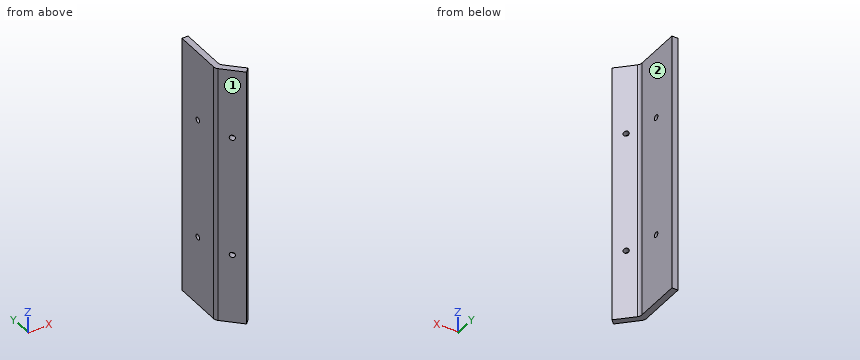
from build123d import *

# Parameters (mm, degrees)
F1_DEPTH = 215
F3_D     = 4.4
F5_D     = 4.4


with BuildPart() as f1:
    # F0 (on Top) → F1 (new body)
    with BuildSketch(Plane.XY):
        with BuildLine():
            Line((0, 2.0710678119), (0, 40))
            Line((0, 40), (-5, 40))
            Line((-5, 40), (-5, 0))
            ThreePointArc((-5, 0), (-4.6193976626, -1.9134171618), (-3.5355339059, -3.5355339059))
            Line((-3.5355339059, -3.5355339059), (10.6066017178, -17.6776695297))
            Line((10.6066017178, -17.6776695297), (14.1421356237, -14.1421356237))
            Line((14.1421356237, -14.1421356237), (1.4644660941, -1.4644660941))
            ThreePointArc((1.4644660941, -1.4644660941), (0.3806023374, 0.15765065), (0, 2.0710678119))
        make_face()
    extrude(amount=F1_DEPTH)

    # F3 (through all)
    with Locations(Plane.YZ):
        with Locations((20, 157.5), (20, 57.5)):
            Hole(F3_D / 2)

    # F5 (through all)
    with Locations(Plane(origin=(0, 0, 0), x_dir=(-0.7071067812, 0.7071067812, 0), z_dir=(0.7071067812, 0.7071067812, 0))):
        with Locations((-10, 157.5), (-10, 57.5)):
            Hole(F5_D / 2)


solid = f1.part
Geometry: final body of the model. Coordinates: model frame, mm. Face numbers are marked on the shaded views. A direction names the side the tool comes from. Round coordinates to 2 decimals unless told otherwise and drop trailing zeros. Loops run counter-clockwise (first coordinate to the right, second up) from the corner with the lowest first, then second, coordinate; pieces in that order, holes last. Notation, with made-up numbers: M 79,61.5 L 107,61.5 A27 cw 107,88.5 Z; hole C 89.25,-22 d9. An arc over 180 degrees is marked long. Put each result on its own line as item: value. Start each with the question number.
(1) Material intervals for line 1 along Z through (x, y) = (-2.6, 20); line 2 along Z through (x, y) = (3.75, -8); line 3 along X through (y, z) = (33, 121), sorted ascending. Write a range as [from, to].
(2) Section query D-D (y = 35.5). Return loops of the section in (x, z), then the cut area to 4 significant figures.
(3) Section query B-B (z = 135.5). Return loops of the section in (x, y).
(4) Contact query for flat-ended pins moving along their axis: pin 1 Ø2 at (x, z) = (6.5, 23.5) entering from -Y; pin 2 Ø1.5 at (x, y) = (-2.5, 6.5) entering from -Z; pin 3 Ø11.5 at (y, z) = (30.5, 135) entering from +X; pin 4 Ø4 at (y, z) = (-3, 179) entering from +X. Output: stop coordinate, or through.
(5) Section query A-A (y = 20). Return loops of the section in (x, z).
(6) Set-up query: the marked faces 1 and 2. Return all of +Z, -Z, +X, -X, +Y, -Y with unobstructed straight access to the full face (end or side cutting, diameter ignored); none if empty.
(7) Section query C-C (z = 157.5). Return loops of the section in (x, y).
Findings below:
1. line 1: z = [0, 55.3], [59.7, 155.3], [159.7, 215]
1. line 2: z = [0, 56.09], [58.91, 156.09], [158.91, 215]
1. line 3: x = [-5, 0]
2. outline: M -5,0 L 0,0 L 0,215 L -5,215 Z
2. area: 1,075 mm2
3. outline: M -5,0 A5 ccw -3.54,-3.54 L 10.61,-17.68 L 14.14,-14.14 L 1.46,-1.46 A5 cw 0,2.07 L 0,40 L -5,40 Z
4. pin 1: stops at y = -14.57
4. pin 2: stops at z = 0
4. pin 3: stops at x = 0
4. pin 4: stops at x = 5
5. outline: M -5,0 L 0,0 L 0,55.3 L -5,55.3 Z; M -5,59.7 L 0,59.7 L 0,155.3 L -5,155.3 Z; M -5,159.7 L 0,159.7 L 0,215 L -5,215 Z
6. face 1: +Z, -Z, -X, -Y
6. face 2: +Z, -Z, +X, +Y
7. outline: M -5,0 A5 ccw -3.54,-3.54 L 1.98,-9.05 L 5.52,-5.52 L 1.46,-1.46 A5 cw 0,2.07 L 0,17.8 L -5,17.8 Z; M -5,22.2 L 0,22.2 L 0,40 L -5,40 Z; M 5.09,-12.16 L 10.61,-17.68 L 14.14,-14.14 L 8.63,-8.63 Z
